from build123d import *

# Parameters (mm, degrees)
F0_W     = 76.2
F0_H     = 88.9
F0_R     = 7.62
F1_DEPTH = 38.1
F2_DEPTH = 19.05
F3_START = -19.05
F3_DEPTH = 19.05
F5_DEPTH = 25.4


with BuildPart() as f1:
    # F0 (on Right) → F1 (new body, symmetric)
    with BuildSketch(Plane.YZ):
        with Locations((0, 19.05)):
            Rectangle(F0_W, F0_H)
        with Locations((0, 26.5176)):
            Circle(F0_R, mode=Mode.SUBTRACT)
    extrude(amount=F1_DEPTH, both=True)

    # F0 (on Right) → F2 (join)
    with BuildSketch(Plane.YZ):
        with BuildLine():
            Line((6.35, -63.5), (38.1, -63.5))
            Line((38.1, -63.5), (38.1, -25.4))
            Line((38.1, -25.4), (-38.1, -25.4))
            Line((-38.1, -25.4), (-38.1, -63.5))
            Line((-38.1, -63.5), (-6.35, -63.5))
            ThreePointArc((-6.35, -63.5), (0, -57.15), (6.35, -63.5))
        make_face()
        with BuildLine():
            ThreePointArc((-38.1, -63.5), (0, -101.6), (38.1, -63.5))
            Line((38.1, -63.5), (6.35, -63.5))
            ThreePointArc((6.35, -63.5), (0, -69.85), (-6.35, -63.5))
            Line((-6.35, -63.5), (-38.1, -63.5))
        make_face()
    extrude(amount=F2_DEPTH)

    # F0 (on Right) → F3 (join)
    with BuildSketch(Plane.YZ.offset(F3_START)):
        with BuildLine():
            Line((6.35, -63.5), (38.1, -63.5))
            Line((38.1, -63.5), (38.1, -25.4))
            Line((38.1, -25.4), (-38.1, -25.4))
            Line((-38.1, -25.4), (-38.1, -63.5))
            Line((-38.1, -63.5), (-6.35, -63.5))
            ThreePointArc((-6.35, -63.5), (0, -57.15), (6.35, -63.5))
        make_face()
        with BuildLine():
            ThreePointArc((-38.1, -63.5), (0, -101.6), (38.1, -63.5))
            Line((38.1, -63.5), (6.35, -63.5))
            ThreePointArc((6.35, -63.5), (0, -69.85), (-6.35, -63.5))
            Line((-6.35, -63.5), (-38.1, -63.5))
        make_face()
    extrude(amount=-F3_DEPTH)

    # F4 (on face) → F5 (cut)
    with BuildSketch(Plane.XY.offset(63.5)):
        with BuildLine():
            ThreePointArc((-30.5689, 32.5501), (-33.9510199549, 33.9510199549), (-32.5501, 30.5689))
            Line((-32.5501, 30.5689), (-32.5501, 32.5501))
            Line((-32.5501, 32.5501), (-30.5689, 32.5501))
        make_face()
        with BuildLine():
            Line((-32.5501, 32.5501), (-32.5501, 30.5689))
            ThreePointArc((-32.5501, 30.5689), (-31.1491800451, 31.1491800451), (-30.5689, 32.5501))
            Line((-30.5689, 32.5501), (-32.5501, 32.5501))
        make_face()
        with BuildLine():
            ThreePointArc((30.5689, 32.5501), (31.1491800451, 31.1491800451), (32.5501, 30.5689))
            Line((32.5501, 30.5689), (32.5501, 32.5501))
            Line((32.5501, 32.5501), (30.5689, 32.5501))
        make_face()
        with BuildLine():
            Line((32.5501, 32.5501), (32.5501, 30.5689))
            ThreePointArc((32.5501, 30.5689), (33.9510199549, 31.1491800451), (34.5313, 32.5501))
            ThreePointArc((34.5313, 32.5501), (32.5501, 34.5313), (30.5689, 32.5501))
            Line((30.5689, 32.5501), (32.5501, 32.5501))
        make_face()
        with BuildLine():
            ThreePointArc((-32.5501, -30.5689), (-33.9510199549, -33.9510199549), (-30.5689, -32.5501))
            Line((-30.5689, -32.5501), (-32.5501, -32.5501))
            Line((-32.5501, -32.5501), (-32.5501, -30.5689))
        make_face()
        with BuildLine():
            Line((-32.5501, -32.5501), (-30.5689, -32.5501))
            ThreePointArc((-30.5689, -32.5501), (-31.1491800451, -31.1491800451), (-32.5501, -30.5689))
            Line((-32.5501, -30.5689), (-32.5501, -32.5501))
        make_face()
        with BuildLine():
            Line((32.5501, -32.5501), (30.5689, -32.5501))
            ThreePointArc((30.5689, -32.5501), (32.5501, -34.5313), (34.5313, -32.5501))
            ThreePointArc((34.5313, -32.5501), (33.9510199549, -31.1491800451), (32.5501, -30.5689))
            Line((32.5501, -30.5689), (32.5501, -32.5501))
        make_face()
        with BuildLine():
            ThreePointArc((32.5501, -30.5689), (31.1491800451, -31.1491800451), (30.5689, -32.5501))
            Line((30.5689, -32.5501), (32.5501, -32.5501))
            Line((32.5501, -32.5501), (32.5501, -30.5689))
        make_face()
    extrude(amount=-F5_DEPTH, mode=Mode.SUBTRACT)


solid = f1.part
Build history of the part. All positions in model axes, mm. A direction names the side the tool comes from. Round coordinates to 2 decimals unless told otherwise and drop trailing zeros. Write each loop counter-clockwise with the first axis right and the second up, starting at its lowest first coordinate (ties: lowest second). Pieces come first, ordered by that corner, then holes. Notation, with made-up numbers: M 1.25,62 L 33.25,62 A27 cw 33.25,89 Z; hole C -21.75,46.5 d11. An arc over 180 degrees is marked long. Answer as a JSON object with one key per item and string values. Group by question number.
(1) Cut at C-C (x = -4.5). Give the cut face in (y, z).
(2) Cut at D-D (x = 4). Give the cut face in (y, z), and give its area (3 significant figures).
(3) Drill centre lines: L1, parallel to Z at x = 13.5, y = 0; L2, parallel to X at y = -28, z = -69; L3, parallel to Y at x = 6.75, z = -63.5. Where is each one in solid material? Low to high.
(4) Cut at B-B (y = 0). Give the cut face in (x, z).
(5) Mould opens along X. For faces 1 (the flat face through (29, -1, -25.4)), 2 (the flat face through (-38.1, -1, -18)), 3 (the flat face through (-19.05, -1, -54)) say: pulls with the +X half, pulls with the -X half, needs draft (parallel to the pull), parting line crosses it, or undercut.
(6) Which spindle directions (+Z, -Z, +X, -X, +Y, -Y) get a long thin tool onto all of the face, cutting with end or side? Do faces 4 (the flat face through (19.05, -1, -54)), 5 (the flat face through (-9, -1, -25.4)), 6 (the flat face through (33, 33, 38.1)). Say none if no direction does.
(7) Flat gauge pins, fed straight in: pin 1 (1.2 mm diameter, centred on x = -32, y = -32, fed in from +Z); pin 2 (5.5 mm diameter, centred on x = -5, y = 16, fed in from -Z); pin 3 (23 mm diameter, centred on y = -7.5, z = -54.5, fed in from +X). Where does each tip first touch, or does it go through?
(8) Cut at A-A (z = -45). Give the cut face in (x, y), and give its area (3 significant figures).
Responses:
{
 "1": {"outline": "M -38.1,-25.4 L 38.1,-25.4 L 38.1,63.5 L -38.1,63.5 Z; hole C 0,26.52 d15.24"},
 "2": {"outline": "M -38.1,-63.5 A38.1 ccw 38.1,-63.5 L 38.1,63.5 L -38.1,63.5 Z; hole C 0,26.52 d15.24; hole C 0,-63.5 d12.7", "area": "11,600 mm2"},
 "3": {"L1": "z = -101.6 to -69.85, -57.15 to 18.9, 34.14 to 63.5", "L2": "x = -38.1 to -19.05, 0 to 19.05", "L3": "y = -38.1 to -6.35, 6.35 to 38.1"},
 "4": {"outline": "M -38.1,-101.6 L -19.05,-101.6 L -19.05,-69.85 L -38.1,-69.85 Z; M -38.1,-57.15 L -19.05,-57.15 L -19.05,-25.4 L 0,-25.4 L 0,-57.15 L 19.05,-57.15 L 19.05,-25.4 L 38.1,-25.4 L 38.1,18.9 L -38.1,18.9 Z; M -38.1,34.14 L 38.1,34.14 L 38.1,63.5 L -38.1,63.5 Z; M 0,-101.6 L 19.05,-101.6 L 19.05,-69.85 L 0,-69.85 Z"},
 "5": {"face 1": "needs draft", "face 2": "pulls with the -X half", "face 3": "undercut"},
 "6": {"face 4": "-Z, +X, +Y, -Y", "face 5": "-Z, +Y, -Y", "face 6": "+Z"},
 "7": {"pin 1": "stops at z = 38.1", "pin 2": "stops at z = -25.4", "pin 3": "stops at x = 19.05"},
 "8": {"outline": "M -38.1,-38.1 L -19.05,-38.1 L -19.05,38.1 L -38.1,38.1 Z; M 0,-38.1 L 19.05,-38.1 L 19.05,38.1 L 0,38.1 Z", "area": "2,900 mm2"}
}
